Input: part model. Units: mm. Frame: model coordinates. Give positions to 0.01 mm unless a question says otherwise; leave off trailing zeros. Order: outer loops, then holes, each group sorted by start corner. A loop starts at its lowest first (then second) coordinate and runs counter-clockwise, first axis right, second up. Notation, with made-up numbers: (28.25, -18) - (33.25, -18) arc R23 ccw to (33.25, 16) - close; hole circle Ø8 at (-12.75, -35). An arc over 180 degrees is marked (long way). Answer in a Markdown table with one row per item. Add a question column.
1. Section query D-D on y = 29. Return loops of the section in (x, z).
2. Contact query for a flat-ended pin moving along its axis: pin 1 (4 mm diameter, centred on x = 80.1, y = 20.34, fed in from -Z) (3 decimals). Output: stop coordinate, or through.
3. Section query A-A on x = 18.62. Return loops of the section in (y, z).
4. Ray query, line 1 (Y direction, x = 18.62, z = 0.8); line 2 (Y direction, x = 80.5, z = 1.2); line 3 (X direction, y = 92.5, z = 0.3). Return the intervals inside material, ascending. Write a range as [from, to].
5. Section query B-B on y = 7.5. Return loops of the section in (x, z).
6. Section query C-C on z = 0.65. Count the separate pieces of the cut face and the enclosed holes in it, and give its area (3 significant figures).
```python
from build123d import *

# Parameters (mm, degrees)
SKETCH_1_R          = 2.1
EXTRUDE_1_DEPTH     = 2
SKETCH_3_R          = 1
CUT_EXTRUDE_1_DEPTH = 10
M4X0_7_1_D          = 3.3
M4X0_7_1_DEPTH      = 11.5
M4X0_7_1_TIP        = 0.991420021


with BuildPart() as part:
    # ｽｹｯﾁ1 → ﾎﾞｽ - 押し出し1 (new body)
    with BuildSketch(Plane.XY):
        Polygon((0, 0), (68.24, 0), (146.992249894, 68.918108191), (146.992249894, 168.01), (0, 168.01), align=None)
        with Locations((18.62, 7.5)):
            Circle(SKETCH_1_R, mode=Mode.SUBTRACT)
        with Locations((48.62, 7.5)):
            Circle(SKETCH_1_R, mode=Mode.SUBTRACT)
        with Locations((139.492249894, 93.468108191)):
            Circle(SKETCH_1_R, mode=Mode.SUBTRACT)
        with Locations((139.492249894, 143.468108191)):
            Circle(SKETCH_1_R, mode=Mode.SUBTRACT)
        with Locations((125.249072144, 59.856479125)):
            Circle(SKETCH_1_R, mode=Mode.SUBTRACT)
        with Locations((80.097280518, 20.342991391)):
            Circle(SKETCH_1_R, mode=Mode.SUBTRACT)
    extrude(amount=EXTRUDE_1_DEPTH)

    # ｽｹｯﾁ3 → ｶｯﾄ - 押し出し1 (cut)
    with BuildSketch(Plane.XY.offset(2)):
        with Locations((10.1, 128.01)):
            Circle(SKETCH_3_R)
        with Locations((30.1, 128.01)):
            Circle(SKETCH_3_R)
        with Locations((120.1, 128.01)):
            Circle(SKETCH_3_R)
    extrude(amount=-CUT_EXTRUDE_1_DEPTH, mode=Mode.SUBTRACT)

    # M4x0.7 ねじ穴1
    with Locations(Plane(origin=(10.1, 128.01, 2), x_dir=(1, 0, 0), z_dir=(0, 0, 1))):
        with Locations((0, 0), (20, 0), (110, 0)):
            Hole(M4X0_7_1_D / 2, depth=M4X0_7_1_DEPTH)
            with Locations((0, 0, -(M4X0_7_1_DEPTH + M4X0_7_1_TIP / 2))):  # 118° drill point
                Cone(0, M4X0_7_1_D / 2, M4X0_7_1_TIP, mode=Mode.SUBTRACT)


solid = part.part
```
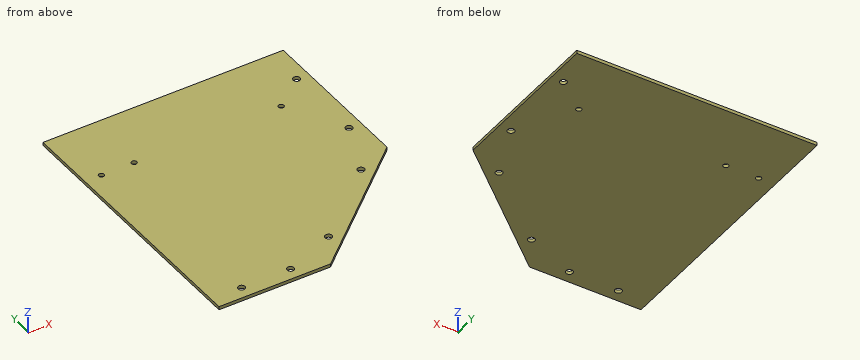
Answer:
| question | item | result |
|---|---|---|
| 1 | outline | (0, 0) - (101.38, 0) - (101.38, 2) - (0, 2) - close |
| 2 | pin 1 | passes through |
| 3 | outline | (0, 0) - (5.4, 0) - (5.4, 2) - (0, 2) - close; (9.6, 0) - (168.01, 0) - (168.01, 2) - (9.6, 2) - close |
| 4 | line 1 | y = [0, 5.4], [9.6, 168.01] |
| 4 | line 2 | y = [10.73, 18.28], [22.4, 168.01] |
| 4 | line 3 | x = [0, 137.63], [141.36, 146.99] |
| 5 | outline | (0, 0) - (16.52, 0) - (16.52, 2) - (0, 2) - close; (20.72, 0) - (46.52, 0) - (46.52, 2) - (20.72, 2) - close; (50.72, 0) - (76.81, 0) - (76.81, 2) - (50.72, 2) - close |
| 6 | separate pieces | 1 |
| 6 | enclosed holes | 9 |
| 6 | area | 21,900 mm² |
